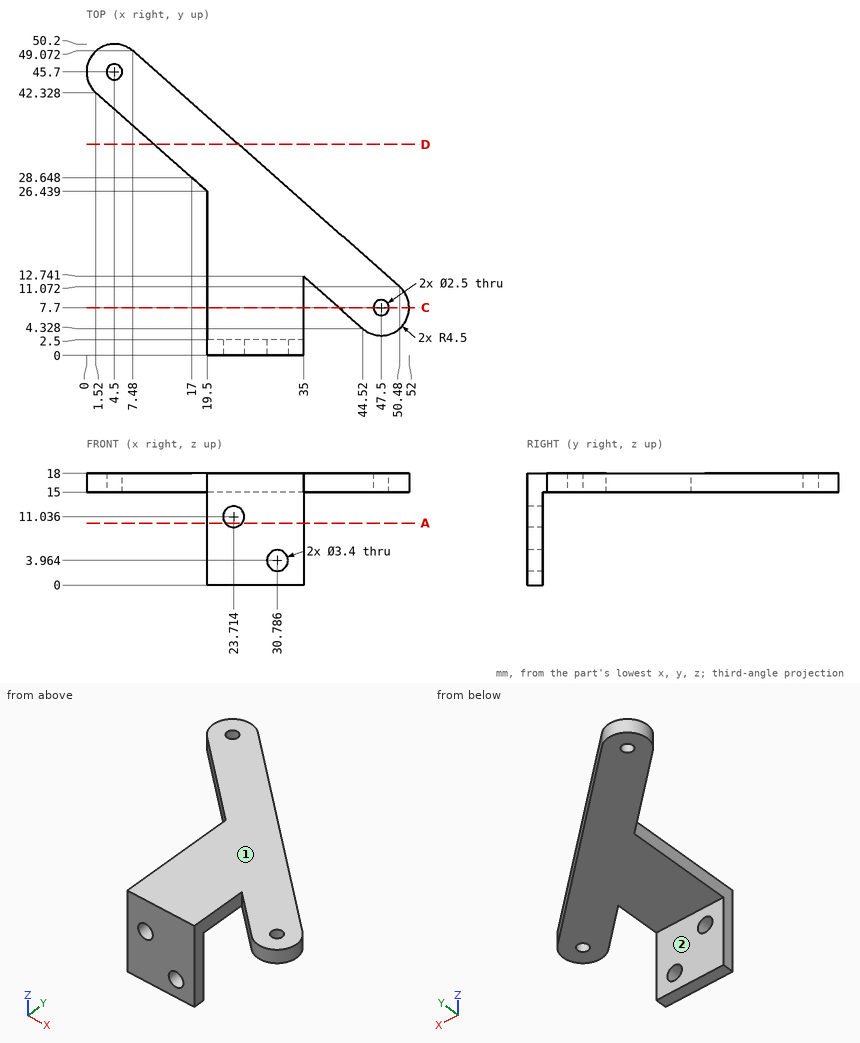
Can you work these out from the drawing? Everything is in mm from the part's minimum corner. A direction names the side the tool comes from. Coordinates: 2 decimals unless noted, no trailing zeros. Loops run counter-clockwise (first coordinate to the right, second up) from the corner with the lowest first, then second, coordinate; pieces in that order, holes last. Notation, with made-up numbers: (-37, -21) - (15, -21) arc R16 ccw to (15, -8) - close; hole circle Ø4 at (71.5, -18.5). An arc over 180 degrees is marked (long way). Answer as CSV lines item,"result".
Q1. If we section it at D-D, the plane y = 34: Write out the boundary of the cut face in (x, z) (1 decimal).
Response:
outline,"(10.9, 15) - (24.5, 15) - (24.5, 18) - (10.9, 18) - close"
Q2. If we section it at A-A, the plane z = 10: Write out the boundary of the cut face in (x, y), and give its area (3 significant figures).
Response:
outline,"(19.5, 0) - (22.37, 0) - (22.37, 2.5) - (19.5, 2.5) - close; (25.06, 0) - (35, 0) - (35, 2.5) - (25.06, 2.5) - close"
area,"32.0 mm2"
Q3. For the marked faces 1 and 2, which set-ups out of +Z, -Z, +X, -X, +Y, -Y let a thin tool reach every point of the face, with its end or its side?
Response:
face 1,"+Z, +X, -X, +Y, -Y"
face 2,"-Z, +X, -X, +Y"
Q4. For pin 1 (4 mm diameter, centred on x = 23.5, z = 11.5, fed in from -Y); pin 2 (1.5 mm diameter, centred on y = 29.5, z = 13.5, fed in from +X); pin 3 (7.5 mm diameter, centred on x = 30.5, z = 5.5, fed in from +Y); pin 4 (3 mm diameter, centred on x = 47.5, y = 7.7, fed in from -Z), each with a flat end and sliding along its axis, tell me the tip position at first contact or that it passes through.
Response:
pin 1,"y = 0"
pin 2,"through"
pin 3,"y = 2.5"
pin 4,"z = 15"
Q5. If we section it at C-C, the plane y = 7.7: Give the number of separate pieces and of enclosed holes in the cut face.
Response:
separate pieces,"3"
enclosed holes,"0"
Q6. If I drill on L1, parallel to Z at x = 32, y = 8; L2, parallel to X at y = 46.5, z = 16; L3, parallel to Y at x = 33.5, z = 7.5, over which ranges is the centre line in solid material (lowest first)? Write a range as [from, to].
Response:
L1,"[15, 18]"
L2,"[0.07, 3.54], [5.46, 10.39]"
L3,"[0, 2.5]"
